```python
from build123d import *

# Parameters (mm, degrees)
SKICA12_R                = 500
P_IDAT_VYSUNUT_M7_DEPTH  = 100
SKICA13_R                = 350
P_IDAT_VYSUNUT_M8_DEPTH  = 100
SKICA14_R                = 200
P_IDAT_VYSUNUT_M9_DEPTH  = 100
SKICA15_R                = 20
P_IDAT_VYSUNUT_M10_DEPTH = 200
P_IDAT_VYSUNUT_M11_DEPTH = 80
P_IDAT_VYSUNUT_M11_TAPER = 56
ZAOBLIT3_R               = 30
ZAOBLIT4_R               = 30
ZAOBLIT5_R               = 20
SKICA21_R                = 35
P_IDAT_VYSUNUT_M12_DEPTH = 250
SKICA22_R                = 460
SKICA22_R_2              = 370
P_IDAT_VYSUNUT_M13_DEPTH = 20
P_IDAT_VYSUNUT_M13_DRAFT = 66


with BuildPart() as part:
    # Skica12 → Přidat vysunutím7 (new body)
    with BuildSketch(Plane.XY):
        Circle(SKICA12_R)
    extrude(amount=P_IDAT_VYSUNUT_M7_DEPTH)

    # Skica13 → Přidat vysunutím8 (add)
    with BuildSketch(Plane.XY.offset(100)):
        Circle(SKICA13_R)
    extrude(amount=P_IDAT_VYSUNUT_M8_DEPTH)

    # Skica14 → Přidat vysunutím9 (add)
    with BuildSketch(Plane.XY.offset(200)):
        Circle(SKICA14_R)
    extrude(amount=P_IDAT_VYSUNUT_M9_DEPTH)

    # Skica15 → Přidat vysunutím10 (add)
    with BuildSketch(Plane.XY.offset(300)):
        with Locations((0, 152.897535665)):
            Circle(SKICA15_R)
        with Locations((132.413150062, 76.448767833)):
            Circle(SKICA15_R)
        with Locations((132.413150062, -76.448767833)):
            Circle(SKICA15_R)
        with Locations((0, -152.897535665)):
            Circle(SKICA15_R)
        with Locations((-132.413150062, -76.448767833)):
            Circle(SKICA15_R)
        with Locations((-132.413150062, 76.448767833)):
            Circle(SKICA15_R)
    extrude(amount=P_IDAT_VYSUNUT_M10_DEPTH)

    # Skica16 → Přidat vysunutím11 (add)
    with BuildSketch(Plane.XY.offset(500)):
        Polygon((-149.73345205, -86.449124779), (0.000412169, -172.897535661), (149.733864218, -86.448410882), (149.73345205, 86.449124779), (-0.000412169, 172.897535661), (-149.733864218, 86.448410882), align=None)
    extrude(amount=P_IDAT_VYSUNUT_M11_DEPTH, taper=P_IDAT_VYSUNUT_M11_TAPER)

    # Zaoblit3
    zaoblit3_edges = [part.edges().sort_by_distance(p)[0] for p in [
        (-500, 0, 100),
    ]]
    fillet(zaoblit3_edges, radius=ZAOBLIT3_R)

    # Zaoblit4
    zaoblit4_edges = [part.edges().sort_by_distance(p)[0] for p in [
        (-350, 0, 200),
    ]]
    fillet(zaoblit4_edges, radius=ZAOBLIT4_R)

    # Zaoblit5
    zaoblit5_edges = [part.edges().sort_by_distance(p)[0] for p in [
        (-200, 0, 300),
    ]]
    fillet(zaoblit5_edges, radius=ZAOBLIT5_R)

    # Skica21 → Přidat vysunutím12 (add)
    with BuildSketch(Plane.XY.offset(100)):
        with Locations((0, 415)):
            Circle(SKICA21_R)
        with Locations((207.5, 359.400542571)):
            Circle(SKICA21_R)
        with Locations((359.400542571, 207.5)):
            Circle(SKICA21_R)
        with Locations((415, 0)):
            Circle(SKICA21_R)
        with Locations((359.400542571, -207.5)):
            Circle(SKICA21_R)
        with Locations((207.5, -359.400542571)):
            Circle(SKICA21_R)
        with Locations((0, -415)):
            Circle(SKICA21_R)
        with Locations((-207.5, -359.400542571)):
            Circle(SKICA21_R)
        with Locations((-359.400542571, -207.5)):
            Circle(SKICA21_R)
        with Locations((-415, 0)):
            Circle(SKICA21_R)
        with Locations((-359.400542571, 207.5)):
            Circle(SKICA21_R)
        with Locations((-207.5, 359.400542571)):
            Circle(SKICA21_R)
    extrude(amount=P_IDAT_VYSUNUT_M12_DEPTH)


with BuildPart() as p_idat_vysunut_m13_tool:
    # Skica22 → Přidat vysunutím13 (with draft: the straight prism first)
    with BuildSketch(Plane.XY.offset(350)):
        Circle(SKICA22_R)
        Circle(SKICA22_R_2, mode=Mode.SUBTRACT)
    extrude(amount=P_IDAT_VYSUNUT_M13_DEPTH)
    # Přidat vysunutím13: the draft: its side faces are tilted about the plane it starts from
    p_idat_vysunut_m13_sides = [p_idat_vysunut_m13_tool.faces().sort_by_distance(p)[0] for p in [
        (-460, 0, 360),
        (-370, 0, 360),
    ]]
    draft(p_idat_vysunut_m13_sides, Plane.XY.offset(350), P_IDAT_VYSUNUT_M13_DRAFT)


with BuildPart() as part_1:
    add(part.part)

    # Přidat vysunutím13: add p_idat_vysunut_m13_tool
    add(p_idat_vysunut_m13_tool.part)


solid = part_1.part
```
Input: part model. Units: mm. Frame: model coordinates. A direction names the side the tool comes from. Coordinates: 2 decimals unless noted, no trailing zeros. Loops run counter-clockwise (first coordinate to the right, second up) from the corner with the lowest first, then second, coordinate; pieces in that order, holes last. Notation, with made-up numbers: (2.25, 71) - (33.25, 71) arc R9 ccw to (33.25, 75) - close; hole circle Ø5 at (60, -25.75). An arc over 180 degrees is marked (long way). Answer in a Markdown table with one row per item.
(1) Set-up query: faces 1 (the face through (-2.604, 172.727, 398.6)), 2 (the face through (-7, 7, 0)), 3 (the face through (-257.96, 236.55, 134.51)). Return all of +Z, -Z, +X, -X, +Y, -Y with unobstructed straight access to the full face (end or side cutting, diameter ignored); none if empty.
Model answer:
| item | result |
|---|---|
| face 1 | none |
| face 2 | -Z, +X, -X, +Y, -Y |
| face 3 | +Z |
(2) Mould query, pull axis Y, two halves, no side actions, for faces 4 (the face through (239.83, -372.81, 223.25)), 5 (the face through (53.27, -89.84, 530.55)), 6 (the face through (-499.516, 21.984, 34.51)). Classes: pulls with the +Y half, pulls with the -Y half, needs draft (parallel to the pull), parting line crosses it, or undercut.
Model answer:
| item | result |
|---|---|
| face 4 | undercut |
| face 5 | pulls with the -Y half |
| face 6 | parting line crosses it |
(3) Cut plane B-B on z = 428.5. Output: boundary loops of the cut face in (x, y), plus the area to 3 significant figures.
Model answer:
| item | result |
|---|---|
| outline | circle Ø40 at (-132.41, -76.45); circle Ø40 at (-132.41, 76.45); circle Ø40 at (0, -152.9); circle Ø40 at (0, 152.9); circle Ø40 at (132.41, -76.45); circle Ø40 at (132.41, 76.45) |
| area | 7,540 mm² |
(4) Pin query (flat end, axial travel): P1, Ø0.8, axis at x = -151, y = -77.5, coming from the +Z side; P2, Ø1, axis at x = 362.5, y = 11.5, coming from the +Z side; P3, Ø8, axis at x = 351.5, z = 340, coming from the +Y side. Return the tip coordinate at first contact, or that it passes through.
Model answer:
| item | result |
|---|---|
| P1 | stops at z = 500 |
| P2 | stops at z = 100 |
| P3 | stops at y = 242.28 |
(5) Material intervals for L1, parallel to X at y = 0.5, z = 271; L2, parallel to Y at x = -391.5, z = 164; L3, parallel to X at y = 229, z = 105, sorted ascending. Write a range as from..to.
Model answer:
| item | result |
|---|---|
| L1 | x = -450..-380, -200..200, 380..450 |
| L2 | y = -221.45..-193.55, -25.94..25.94, 193.55..221.45 |
| L3 | x = -387.02..-331.78, -264.69..264.69, 331.78..387.02 |
(6) Cut plane A-A on z = 322. Count the separate pieces of the cut face and the enclosed holes in it, plus the area to 3 significant figures.
Model answer:
| item | result |
|---|---|
| separate pieces | 18 |
| enclosed holes | 0 |
| area | 53,700 mm² |
